Geometry check sheet. Reference: the model listing, model coordinates, mm. A direction names the side the tool comes from. Give positions to 0.01 mm unless a question says otherwise; leave off trailing zeros. Loops run counter-clockwise (first coordinate to the right, second up) from the corner with the lowest first, then second, coordinate; pieces in that order, holes last. Notation, with made-up numbers: (-39.5, -16.5) - (-30.5, -16.5) arc R19 ccw to (-30.5, 17.5) - close; hole circle Ø9 at (43, 59). An arc over 180 degrees is marked (long way). Use a Markdown table: item, result. Add a question column.
1. Cross-section at C-C on x = 0. Enter the section's corners in (y, z).
2. Draft check along Z on faces 4 (the cylindrical face through (0.156, 25.026, 4.649)), 5 (the flat face through (-0.2, 8.8, 4.775)), 6 (the flat face through (11.112, 13, 13)). Enter one of: pulls with the +Z half, pulls with the -Z half, needs draft (parallel to the pull), parting line crosses it, or undercut.
3. Cross-section at B-B on z = 17.5. Enter the section's corners in (x, y), and give its area (3 significant figures).
4. Cross-section at A-A on x = -7. Enter the section's corners in (y, z).
5. Set-up check for faces 1 (the flat face through (-3, 16, 0)), 2 (the cylindrical face through (0.86, 18.99, 6.08)), 3 (the cylindrical face through (-0.86, 6.08, 18.99)): record each of +Z, -Z, +X, -X, +Y, -Y from which the full face is reachable in a straight line by a thin tool's end or side.
6. Depth check by flat-ended pin: P1, Ø8, axis at x = -7.5, z = 12, coming from the +Y side; P2, Ø10, axis at x = 7.5, z = 10, coming from the +Y side; P3, Ø4.5, axis at x = -2, z = 8.5, coming from the +Y side. Enter the tip coordinate at first touch or a pass-through.
7. Material ranges on L1, parallel to Y at x = 0, z = 1; L2, parallel to X at y = 16.75, z = 12.5; L3, parallel to X at y = 2.7, z = 12.7, recorded low to high.
8. Cross-section at D-D on y = 7.5. Enter the section's corners in (x, z).
from build123d import *

# Parameters (mm, degrees)
BOSS_EXTRUDE1_START      = -11.1125
BOSS_EXTRUDE1_DEPTH      = 22.225
BOSS_EXTRUDE1_START_2    = 4.7752
BOSS_EXTRUDE1_2_DEPTH    = 20.6248
BOSS_EXTRUDE1_START_3    = 4
BOSS_EXTRUDE1_3_DEPTH    = 21.4
SKETCH2_W                = 22.225
SKETCH2_H                = 25.4
BOSS_EXTRUDE2_DEPTH      = 4.7752
K_0_281_DIAMETER_HOLE1_D = 7.1374
K_0_281_DIAMETER_HOLE2_D = 7.1374
FILLET1_R                = 4.7752


with BuildPart() as part:
    # Boss-Extrude1: read off the stored shape, not the designer's step
    # Boss-Extrude1 outline → Boss-Extrude1 (new body)
    with BuildSketch(Plane.YZ.offset(BOSS_EXTRUDE1_START)):
        Polygon((25.4, 4.7752), (4.7752, 25.4), (4.7752, 18.646847397), (18.646847397, 4.7752), (4.7752, 4.7752), (4.7752, 0), (25.4, 0), align=None)
    extrude(amount=BOSS_EXTRUDE1_DEPTH)

    # Boss-Extrude1 2 outline → Boss-Extrude1 2 (cut)
    with BuildSketch(Plane.XY.offset(BOSS_EXTRUDE1_START_2)):
        with BuildLine():
            ThreePointArc((6.272513521, 11.711023698), (0, 19.05), (-6.272513521, 11.711023698))
            ThreePointArc((-6.272513521, 11.711023698), (0, 6.35), (6.272513521, 11.711023698))
        make_face()
    extrude(amount=BOSS_EXTRUDE1_2_DEPTH, mode=Mode.SUBTRACT)

    # Boss-Extrude1 3 outline → Boss-Extrude1 3 (cut)
    with BuildSketch(Plane(origin=(0, 0, 0), x_dir=(1, 0, 0), z_dir=(0, 1, 0)).offset(BOSS_EXTRUDE1_START_3)):
        with BuildLine():
            ThreePointArc((-6.272513521, -11.711023698), (0, -19.05), (6.272513521, -11.711023698))
            ThreePointArc((6.272513521, -11.711023698), (0, -6.35), (-6.272513521, -11.711023698))
        make_face()
    extrude(amount=BOSS_EXTRUDE1_3_DEPTH, mode=Mode.SUBTRACT)

    # Sketch2 → Boss-Extrude2 (add)
    with BuildSketch(Plane.XZ.offset(-4.7752)):
        with Locations((0, 12.7)):
            Rectangle(SKETCH2_W, SKETCH2_H)
    extrude(amount=BOSS_EXTRUDE2_DEPTH)

    # K (0.281) Diameter Hole1 (through all)
    with Locations(Plane(origin=(0, 0, 0), x_dir=(-1, 0, 0), z_dir=(0, -1, 0))):
        with Locations((0, -12.7)):
            Hole(K_0_281_DIAMETER_HOLE1_D / 2)

    # K (0.281) Diameter Hole2 (through all)
    with Locations(Plane.XY.offset(4.7752)):
        with Locations((0, 12.7)):
            Hole(K_0_281_DIAMETER_HOLE2_D / 2)

    # Fillet1
    fillet1_edges = [part.edges().sort_by_distance(p)[0] for p in [
        (0, 25.4, 4.7752),
        (0, 4.7752, 25.4),
    ]]
    fillet(fillet1_edges, radius=FILLET1_R)


solid = part.part
Values found:
| question | item | result |
|---|---|---|
| 1 | outline | (0, 0) - (9.13, 0) - (9.13, 4.78) - (4.78, 4.78) - (4.78, 9.13) - (0, 9.13) - close; (0, 16.27) - (4.78, 16.27) - (4.78, 19.05) - (6.35, 19.05) - (6.35, 23.83) - (6.17, 24) arc R4.78 ccw to (2.8, 25.4) - (0, 25.4) - close; (16.27, 0) - (25.4, 0) - (25.4, 2.8) arc R4.78 ccw to (24, 6.17) - (23.83, 6.35) - (19.05, 6.35) - (19.05, 4.78) - (16.27, 4.78) - close |
| 2 | face 4 | pulls with the +Z half |
| 2 | face 5 | undercut |
| 2 | face 6 | needs draft |
| 3 | outline | (-11.11, 0) - (11.11, 0) - (11.11, 4.78) - (-11.11, 4.78) - close; (-11.11, 5.92) - (-4.16, 5.92) - (-4.16, 7.9) arc R6.35 cw to (-6.35, 12.68) - (-11.11, 12.68) - close; (4.16, 5.92) - (11.11, 5.92) - (11.11, 12.68) - (6.35, 12.68) arc R6.35 cw to (4.16, 7.9) - close |
| 3 | area | 186 mm2 |
| 4 | outline | (0, 0) - (25.4, 0) - (25.4, 2.8) arc R4.78 ccw to (24, 6.17) - (6.17, 24) arc R4.78 ccw to (2.8, 25.4) - (0, 25.4) - close; hole (4.78, 4.78) - (18.65, 4.78) - (4.78, 18.65) - close |
| 5 | face 1 | -Z, +X, -X, +Y, -Y |
| 5 | face 2 | +Z |
| 5 | face 3 | +Y |
| 6 | P1 | stops at y = 22.18 |
| 6 | P2 | stops at y = 24.86 |
| 6 | P3 | stops at y = 23.93 |
| 7 | L1 | y = 0 to 9.13, 16.27 to 25.4 |
| 7 | L2 | x = -11.11 to -6.35, 6.35 to 11.11 |
| 7 | L3 | x = -11.11 to -3.57, 3.57 to 11.11 |
| 8 | outline | (-11.11, 0) - (11.11, 0) - (11.11, 4.78) - (-11.11, 4.78) - close; (-11.11, 15.92) - (-5.47, 15.92) arc R6.35 cw to (-3.64, 17.9) - (-3.64, 22.68) - (-11.11, 22.68) - close; (3.64, 17.9) arc R6.35 cw to (5.47, 15.92) - (11.11, 15.92) - (11.11, 22.68) - (3.64, 22.68) - close |
